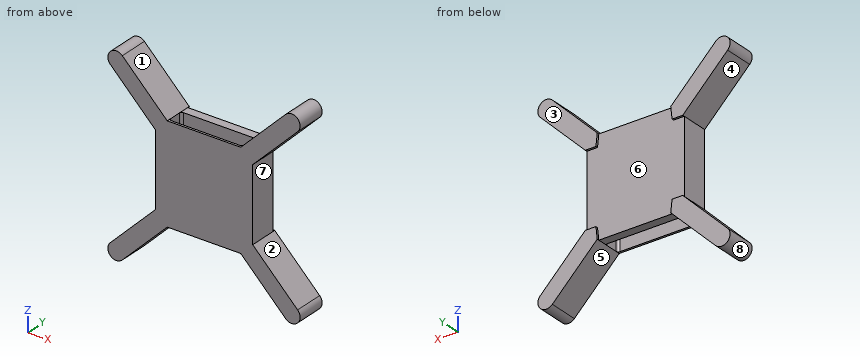
```python
from build123d import *

# Parameters (mm, degrees)
SKETCH1_W           = 46
SKETCH1_H           = 46
BOSS_EXTRUDE1_DEPTH = 13
CUT_EXTRUDE2_DEPTH  = 10
BOSS_EXTRUDE2_START = -13
BOSS_EXTRUDE2_DEPTH = 14
CUT_EXTRUDE4_DEPTH  = 63


# Read off the part's stored shape, not the designer's step: Boss-Extrude2
with BuildPart() as part:
    # Sketch1 → Boss-Extrude1 (new body)
    with BuildSketch(Plane(origin=(0, 0, 0), x_dir=(1, 0, 0), z_dir=(0, 1, 0))):
        Rectangle(SKETCH1_W, SKETCH1_H)
    extrude(amount=BOSS_EXTRUDE1_DEPTH)

    # Sketch2 → Cut-Extrude2 (cut)
    with BuildSketch(Plane(origin=(0, 13, 0), x_dir=(1, 0, 0), z_dir=(0, 1, 0))):
        Polygon((17.339375574, 23), (17.969631493, 17.346908404), (23, 17.346908404), (23, 23), align=None)
        Polygon((-23, 23), (-17.339375574, 23), (-17.969631493, 17.346908404), (-23, 17.346908404), align=None)
        Polygon((-23, -17.346908404), (-23, -23), (-17.339375574, -23), (-17.969631493, -17.346908404), align=None)
        Polygon((17.339375574, -23), (23, -23), (23, -17.346908404), (17.969631493, -17.346908404), align=None)
    extrude(amount=-CUT_EXTRUDE2_DEPTH, mode=Mode.SUBTRACT)

    # Boss-Extrude2 outline → Boss-Extrude2 (add)
    with BuildSketch(Plane(origin=(0, 13, 0), x_dir=(1, 0, 0), z_dir=(0, 1, 0)).offset(BOSS_EXTRUDE2_START)):
        with BuildLine():
            Line((-38.538452146, -44.227320898), (-17.339375574, -23))
            Line((-17.339375574, -23), (-17.969631493, -17.346908404))
            Line((-17.969631493, -17.346908404), (-23, -17.346908404))
            Line((-23, -17.346908404), (-44.202839223, -38.577999476))
            ThreePointArc((-44.202839223, -38.577999476), (-44.195306563, -44.234853893), (-38.538452146, -44.227320898))
        make_face()
        with BuildLine():
            Line((-17.969631493, 17.346908404), (-17.339375574, 23))
            Line((-17.339375574, 23), (-38.538452146, 44.227320898))
            ThreePointArc((-38.538452146, 44.227320898), (-44.195306563, 44.234853893), (-44.202839223, 38.577999476))
            Line((-44.202839223, 38.577999476), (-23, 17.346908404))
            Line((-23, 17.346908404), (-17.969631493, 17.346908404))
        make_face()
        with BuildLine():
            Line((44.202839223, -38.577999476), (23, -17.346908404))
            Line((23, -17.346908404), (17.969631493, -17.346908404))
            Line((17.969631493, -17.346908404), (17.339375574, -23))
            Line((17.339375574, -23), (38.538452146, -44.227320898))
            ThreePointArc((38.538452146, -44.227320898), (44.195306563, -44.234853893), (44.202839223, -38.577999476))
        make_face()
        with BuildLine():
            Line((17.969631493, 17.346908404), (23, 17.346908404))
            Line((23, 17.346908404), (44.202839223, 38.577999476))
            ThreePointArc((44.202839223, 38.577999476), (44.195306563, 44.234853893), (38.538452146, 44.227320898))
            Line((38.538452146, 44.227320898), (17.339375574, 23))
            Line((17.339375574, 23), (17.969631493, 17.346908404))
        make_face()
    extrude(amount=BOSS_EXTRUDE2_DEPTH)

    # Sketch5 → Cut-Extrude4 (cut)
    with BuildSketch(Plane.XY.offset(23)):
        with BuildLine():
            Line((-16.339375574, 1), (16.339375574, 1))
            ThreePointArc((16.339375574, 1), (17.046482355, 1.292893219), (17.339375574, 2))
            Line((17.339375574, 2), (17.339375574, 7.824688375))
            ThreePointArc((17.339375574, 7.824688375), (17.046482355, 8.531795157), (16.339375574, 8.824688375))
            Line((16.339375574, 8.824688375), (-16.339375574, 8.824688375))
            ThreePointArc((-16.339375574, 8.824688375), (-17.046482355, 8.531795157), (-17.339375574, 7.824688375))
            Line((-17.339375574, 7.824688375), (-17.339375574, 2))
            ThreePointArc((-17.339375574, 2), (-17.046482355, 1.292893219), (-16.339375574, 1))
        make_face()
    extrude(amount=-CUT_EXTRUDE4_DEPTH, mode=Mode.SUBTRACT)


solid = part.part
```
The model under review builds one solid part; all positions refer to its coordinate system, in mm. Face numbers are marked on the shaded views. A direction names the side the tool comes from. Round coordinates to 2 decimals unless told otherwise and drop trailing zeros. Write each loop counter-clockwise with the first axis right and the second up, starting at its lowest first coordinate (ties: lowest second). Pieces come first, ordered by that corner, then holes.
(1) We need section D-D on y = 11. Give the boundary of the cut face in (x, z), and give its area (3 significant figures).
(2) We need section B-B on y = 4.75. Give the boundary of the cut face in (x, z).
(3) Mouldability with a two-part tool opening along Z and no side actions: class the marked faces 1, 2 and 3 as +Z half, -Z half, draft (parallel to the pull), parting line (faces both ways), or undercut.
(4) Insertion check: pin 1 (0.5 mm diameter, centred on x = 20.5, y = 13.5, fed in from +Z); pin 2 (3 mm diameter, centred on y = 5.5, z = -18.5, fed in from +X); pin 3 (1.6 mm diameter, centred on x = 6.5, y = 11.5, fed in from -Z); pin 4 (8 mm diameter, centred on x = 22, z = -27, fed in from -Y). Each pin has a flat end and moves straight along its axis. Give the tip position at first contact, or say it passes through.
(5) Wall thickness on L1, parallel to X at y = 6.5, z = 14.5; L2, parallel to Y at x = -8, z = 4; L3, parallel to Z at x = -30.5, y = 12.5: over which ranges is each line inside the solid? List them lowest first.
(6) Machinability: for the marked faces 4, 5, 6, 7 and 8, which of the approach directions +Z, -Z, +X, -X, +Y, -Y give a long, thin tool a straight path to every point of the face, cutting with its end or side? Answer none if there is none.
(7) We need section C-C on z = 10. Give the boundary of the cut face in (x, y).
(8) We need section A-A on x = -7. Give the boundary of the cut face in (y, z).
Findings below:
1. outline: (-44.2, -38.58) arc R4 ccw to (-38.54, -44.23) - (-17.34, -23) - (17.34, -23) - (38.54, -44.23) arc R4 ccw to (44.2, -38.58) - (23, -17.35) - (23, 17.35) - (44.2, 38.58) arc R4 ccw to (38.54, 44.23) - (17.34, 23) - (-17.34, 23) - (-38.54, 44.23) arc R4 ccw to (-44.2, 38.58) - (-23, 17.35) - (-23, -17.35) - close
1. area: 3,110 mm2
2. outline: (-44.2, -38.58) arc R4 ccw to (-38.54, -44.23) - (-17.34, -23) - (-17.34, 23) - (-38.54, 44.23) arc R4 ccw to (-44.2, 38.58) - (-23, 17.35) - (-23, -17.35) - close; (17.34, -23) - (38.54, -44.23) arc R4 ccw to (44.2, -38.58) - (23, -17.35) - (23, 17.35) - (44.2, 38.58) arc R4 ccw to (38.54, 44.23) - (17.34, 23) - close
3. face 1: +Z half
3. face 2: undercut
3. face 3: draft
4. pin 1: stops at z = 26.42
4. pin 2: stops at x = 25.65
4. pin 3: stops at z = -23
4. pin 4: stops at y = 0
5. L1: x = -23 to -17.34, 17.34 to 23
5. L2: y = 0 to 1, 8.82 to 13
5. L3: z = -36.18 to -24.86, 24.86 to 36.18
6. face 4: -X, +Y, -Y
6. face 5: -Z, +Y, -Y
6. face 6: +Y
6. face 7: +X, +Y, -Y
6. face 8: +Y, -Y
7. outline: (-23, 0) - (23, 0) - (23, 13) - (-23, 13) - close; hole (-17.34, 2) arc R1 ccw to (-16.34, 1) - (16.34, 1) arc R1 ccw to (17.34, 2) - (17.34, 7.82) arc R1 ccw to (16.34, 8.82) - (-16.34, 8.82) arc R1 ccw to (-17.34, 7.82) - close
8. outline: (0, -23) - (1, -23) - (1, 23) - (0, 23) - close; (8.82, -23) - (13, -23) - (13, 23) - (8.82, 23) - close
